Model file for the job. Use its own axes, mm. A direction names the side the tool comes from. Give positions to 0.01 mm unless a question says otherwise; leave off trailing zeros. Order: outer loops, then holes, each group sorted by start corner. A loop starts at its lowest first (then second) coordinate and runs counter-clockwise, first axis right, second up. Notation, with made-up numbers: (79.5, 62) - (85.5, 62) arc R28 ccw to (85.5, 89) - close; hole circle Ø1 at (-16.75, -3). An arc over 180 degrees is marked (long way). Return JSON: item names as keys, results as strings. Group by question number.
from build123d import *

# Parameters (mm, degrees)
BOSS_EXTRUDE1_DEPTH = 170
SKETCH2_R           = 2.75
CUT_EXTRUDE1_DEPTH  = 9
SKETCH3_R           = 1.7
CUT_EXTRUDE2_DEPTH  = 9
SKETCH4_R           = 3.375
CUT_EXTRUDE3_DEPTH  = 3.5
FILLET1_R           = 3
SKETCH5_R           = 27.5
CUT_EXTRUDE4_DEPTH  = 9
FILLET2_R           = 3
FILLET3_R           = 3
SKETCH6_W           = 170
SKETCH6_H           = 25
CUT_EXTRUDE5_DEPTH  = 9
FILLET4_R           = 3
FILLET5_R           = 3


with BuildPart() as part:
    # Sketch1 → Boss-Extrude1 (new body)
    with BuildSketch(Plane.XY):
        Polygon((-85, 0), (0, 0), (85, 0), (85, -8), (-85, -8), align=None)
    extrude(amount=-BOSS_EXTRUDE1_DEPTH)

    # Sketch2 → Cut-Extrude1 (cut, through all)
    with BuildSketch(Plane(origin=(0, 0, 0), x_dir=(1, 0, 0), z_dir=(0, 1, 0))):
        with Locations((-75, 35)):
            Circle(SKETCH2_R)
        with Locations((75, 35)):
            Circle(SKETCH2_R)
        with Locations((75, 135)):
            Circle(SKETCH2_R)
        with Locations((-75, 135)):
            Circle(SKETCH2_R)
    extrude(amount=-CUT_EXTRUDE1_DEPTH, mode=Mode.SUBTRACT)

    # Sketch3 → Cut-Extrude2 (cut, through all)
    with BuildSketch(Plane(origin=(0, 0, 0), x_dir=(1, 0, 0), z_dir=(0, 1, 0))):
        with Locations((-45.35, 45.25)):
            Circle(SKETCH3_R)
        with Locations((46.25, 45.25)):
            Circle(SKETCH3_R)
        with Locations((46.25, 123.75)):
            Circle(SKETCH3_R)
        with Locations((-45.35, 123.75)):
            Circle(SKETCH3_R)
    extrude(amount=-CUT_EXTRUDE2_DEPTH, mode=Mode.SUBTRACT)

    # Sketch4 → Cut-Extrude3 (cut)
    with BuildSketch(Plane.XZ.offset(8)):
        with Locations((-45.35, -45.25)):
            Circle(SKETCH4_R)
        with Locations((46.25, -45.25)):
            Circle(SKETCH4_R)
        with Locations((46.25, -123.75)):
            Circle(SKETCH4_R)
        with Locations((-45.35, -123.75)):
            Circle(SKETCH4_R)
    extrude(amount=-CUT_EXTRUDE3_DEPTH, mode=Mode.SUBTRACT)

    # Fillet1
    fillet1_edges = [part.edges().sort_by_distance(p)[0] for p in [
        (0, 0, -170),
        (0, 0, 0),
        (-85, 0, -85),
        (85, 0, -85),
    ]]
    fillet(fillet1_edges, radius=FILLET1_R)

    # Sketch5 → Cut-Extrude4 (cut, through all)
    with BuildSketch(Plane(origin=(0, 0, 0), x_dir=(1, 0, 0), z_dir=(0, 1, 0))):
        with Locations((-0.5, 85.5)):
            Circle(SKETCH5_R)
    extrude(amount=-CUT_EXTRUDE4_DEPTH, mode=Mode.SUBTRACT)

    # Fillet2
    fillet2_edges = [part.edges().sort_by_distance(p)[0] for p in [
        (-28, 0, -85.5),
    ]]
    fillet(fillet2_edges, radius=FILLET2_R)

    # Fillet3
    fillet3_edges = [part.edges().sort_by_distance(p)[0] for p in [
        (-28, -8, -85.5),
    ]]
    fillet(fillet3_edges, radius=FILLET3_R)

    # Sketch6 → Cut-Extrude5 (cut, through all)
    with BuildSketch(Plane(origin=(0, 0, 0), x_dir=(1, 0, 0), z_dir=(0, 1, 0))):
        with Locations((0, 157.5)):
            Rectangle(SKETCH6_W, SKETCH6_H)
        with Locations((0, 12.5)):
            Rectangle(SKETCH6_W, SKETCH6_H)
    extrude(amount=-CUT_EXTRUDE5_DEPTH, mode=Mode.SUBTRACT)

    # Fillet4
    fillet4_edges = [part.edges().sort_by_distance(p)[0] for p in [
        (0, 0, -145),
        (-85, -5.5, -145),
        (85, -5.5, -145),
    ]]
    fillet(fillet4_edges, radius=FILLET4_R)

    # Fillet5
    fillet5_edges = [part.edges().sort_by_distance(p)[0] for p in [
        (85, -5.5, -25),
        (-85, -5.5, -25),
        (0, 0, -25),
    ]]
    fillet(fillet5_edges, radius=FILLET5_R)


solid = part.part
(1) Drop a flat-ended pin along its axis: pin 1 Ø2 at (x, z) = (-45, -44) entering from -Y. Give the stop position or say it passes through.
(2) Slice it at A-A (z = -45.25). Give the cut face in (x, y) (3 decimals).
(3) Slice it at C-C (x = -75). Give the cut face in (y, z), and give its area (3 significant figures).
(4) Slice it at D-D (z = -135). Give the cut face in (x, y), and give its area (3 significant figures).
(5) Pull direction Z, two halves, no side cores. Call faces 1 (the face through (45, -4.5, -122)), 2 (the face through (-17, 0, -59)), 3 (the face through (-1, -5, -145)): released by +Z, released by -Z, zero draft, split by the parting line, or undercut.
(6) Drill centre lines: L1, parallel to X at y = -6.5, z = -35; L2, parallel to Z at x = -45.35, y = -5.75 (3 decimals); L3, parallel to Z at x = 75, y = -1.75. Where is each one in solid material? Low to high.
(7) 3-axis set-ups, long thin cutter, end or side, ignore diameter. For faces 4 (the face through (-46, -4.5, -122)), 5 (the face through (-1, -5, -25)): which of +Z, -Z, +X, -X, +Y, -Y reach the whole face in a straight line?
(8) Slice it at B-B (x = -0.5). Give the cut face in (y, z), and give its area (3 significant figures).
Result set:
{
 "1": {"pin 1": "stops at y = -4.5"},
 "2": {"outline": "(-85, -8) - (-48.725, -8) - (-48.725, -4.5) - (-47.05, -4.5) - (-47.05, 0) - (-82, 0) arc R3 ccw to (-85, -3) - close; (-43.65, -4.5) - (-41.975, -4.5) - (-41.975, -8) - (42.875, -8) - (42.875, -4.5) - (44.55, -4.5) - (44.55, 0) - (-43.65, 0) - close; (47.95, -4.5) - (49.625, -4.5) - (49.625, -8) - (85, -8) - (85, -3) arc R3 ccw to (82, 0) - (47.95, 0) - close"},
 "3": {"outline": "(-8, -145) - (-3, -145) arc R3 ccw to (0, -142) - (0, -137.75) - (-8, -137.75) - close; (-8, -132.25) - (0, -132.25) - (0, -37.75) - (-8, -37.75) - close; (-8, -32.25) - (0, -32.25) - (0, -28) arc R3 ccw to (-3, -25) - (-8, -25) - close", "area": "868 mm²"},
 "4": {"outline": "(-85, -8) - (-77.75, -8) - (-77.75, 0) - (-82, 0) arc R3 ccw to (-85, -3) - close; (-72.25, -8) - (72.25, -8) - (72.25, 0) - (-72.25, 0) - close; (77.75, -8) - (85, -8) - (85, -3) arc R3 ccw to (82, 0) - (77.75, 0) - close", "area": "1,270 mm²"},
 "5": {"face 1": "undercut", "face 2": "zero draft", "face 3": "released by -Z"},
 "6": {"L1": "x = -85 to -77.75, -72.25 to 72.25, 77.75 to 85", "L2": "z = -145 to -127.125, -120.375 to -48.625, -41.875 to -25", "L3": "z = -144.73 to -137.75, -132.25 to -37.75, -32.25 to -25.27"},
 "7": {"face 4": "-Y", "face 5": "+Z, +X, -X, +Y, -Y"},
 "8": {"outline": "(-8, -145) - (-3, -145) arc R3 ccw to (0, -142) - (0, -116) arc R3 ccw to (-3, -113) - (-5, -113) arc R3 ccw to (-8, -116) - close; (-8, -55) arc R3 ccw to (-5, -58) - (-3, -58) arc R3 ccw to (0, -55) - (0, -28) arc R3 ccw to (-3, -25) - (-8, -25) - close", "area": "508 mm²"}
}
